Design review of the part built by this model. Coordinates are the model's own, in mm. Face numbers are marked on the shaded views. A direction names the side the tool comes from. Give positions to 0.01 mm unless a question says otherwise; leave off trailing zeros. Write each loop counter-clockwise with the first axis right and the second up, starting at its lowest first coordinate (ties: lowest second). Pieces come first, ordered by that corner, then holes. Notation, with made-up numbers: M 88,18.25 L 129,18.25 A35 ccw 129,56.25 Z; hole C 5.5,-5.5 d1. An arc over 180 degrees is marked long. One line per item, written item: value. Start each with the question number.
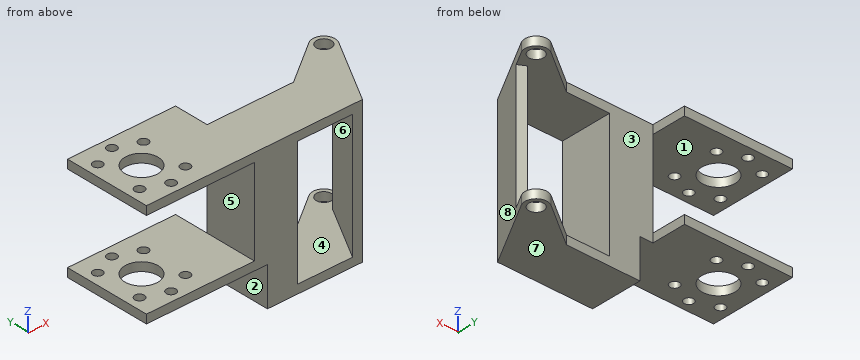
Autodesk Inventor part; units mm, degrees
ref_plane "YZ Plane" through (0, 0, 0) normal (1, 0, 0) x (0, 1, 0)
ref_plane "XZ Plane" through (0, 0, 0) normal (0, 1, 0) x (-1, 0, 0)
ref_plane "XY Plane" through (0, 0, 0) normal (0, 0, 1) x (1, 0, 0)
sketch "Sketch1" plane through (0, 0, 0) normal (0, 1, 0) x (-1, 0, 0)
  line L0 (10.16, 20.955) -> (-21.59, 20.955)
  line L1 (-21.59, 20.955) -> (-21.59, 18.415)
  line L2 (-21.59, 18.415) -> (10.16, 18.415)
  line L3 (10.16, 18.415) -> (10.16, 20.955)
  line L4 (10.16, -6.985) -> (-21.59, -6.985)
  line L5 (-21.59, -6.985) -> (-21.59, -9.525)
  line L6 (-21.59, -9.525) -> (10.16, -9.525)
  line L7 (10.16, -9.525) -> (10.16, -6.985)
  point P0 (0, 0)
  dimension "d0" = 31.75
  dimension "d1" = 2.54
  dimension "d2" = 10.16
  dimension "d3" = 20.955
  dimension "d4" = 31.75
  dimension "d5" = 2.54
  dimension "d6" = 10.16
  dimension "d7" = 30.48
extrude "Extrusion1" add sketch "Sketch1" along normal blind 25.4
sketch "Sketch2" plane through (0, 0, 0) normal (0, 1, 0) x (-1, 0, 0)
  line L0 (-21.59, 18.415) -> (10.16, 18.415)
  line L1 (10.16, -6.985) -> (-21.59, -6.985)
  line L2 (-21.59, 18.415) -> (-34.29, 18.415)
  line L3 (10.16, 18.415) -> (10.16, 20.955)
  line L4 (-21.59, -9.525) -> (-25.4, -9.525)
  line L5 (-21.59, -6.985) -> (-21.59, -9.525)
  line L6 (-21.59, -9.525) -> (-21.59, 18.415)
  line L7 (-25.4, -9.525) -> (-25.4, -20.955)
  line L8 (-25.4, -20.955) -> (-34.29, -20.955)
  line L9 (-34.29, -20.955) -> (-34.29, 18.415)
  line L10 (-21.59, 18.415) -> (10.16, 18.415)
  line L11 (10.16, -9.525) -> (10.16, -6.985)
  line L12 (10.16, 20.955) -> (-21.59, 20.955)
  point P0 (0, 0)
  point P1 (-21.59, -6.985)
  dimension "d16" = 35.56
  dimension "d17" = 41.91
  dimension "d18" = 12.7
extrude "Extrusion2" add sketch "Sketch2" along normal blind 15.24
sketch "Sketch4" plane through (0, 0, 0) normal (0, 1, 0) x (-1, 0, 0)
  line L0 (-34.29, -20.955) -> (-25.4, -20.955)
  line L1 (-34.29, -20.955) -> (-53.34, -20.955)
  line L2 (-53.34, -20.955) -> (-53.34, -18.415)
  line L3 (-53.34, -18.415) -> (-34.29, -18.415)
  line L4 (-34.29, -18.415) -> (-34.29, -20.955)
  line L5 (-21.59, 20.955) -> (-53.34, 20.955)
  line L6 (-53.34, 20.955) -> (-53.34, 18.415)
  line L7 (-53.34, 18.415) -> (-21.59, 18.415)
  line L8 (-21.59, 18.415) -> (-21.59, 20.955)
  line L9 (10.16, 18.415) -> (10.16, 20.955)
  line L10 (10.16, -9.525) -> (10.16, -6.985)
  point P0 (0, 0)
  point P1 (-50.8, -18.415)
  dimension "d20" = 2.54
  dimension "d24" = 2.54
  dimension "d55" = 63.5
  dimension "d56" = 63.5
extrude "Extrusion3" add sketch "Sketch4" along normal blind 15.24
sketch "Sketch5" plane through (-10.16, 25.4, 20.955) normal (0, 0, 1) x (1, 0, 0)
  circle A0 centre (10.16, -12.7) radius 4.8895
  line L0 (0, -25.4) -> (0, 0)
  line L1 (-16.3, -25.4) -> (92.4658, -25.4)
  circle A1 centre (10.16, -22.225) radius 1.397
  circle A2 centre (16.8952, -19.4352) radius 1.397
  circle A3 centre (19.685, -12.7) radius 1.397
  circle A4 centre (16.8952, -5.9648) radius 1.397
  circle A5 centre (10.16, -3.175) radius 1.397
  circle A6 centre (3.4248, -5.9648) radius 1.397
  circle A7 centre (0.635, -12.7) radius 1.397
  circle A8 centre (3.4248, -19.4352) radius 1.397
  point P0 (10.16, -25.4)
  dimension "d26" = 9.779
  dimension "d27" = 10.16
  dimension "d28" = 12.7
  dimension "d29" = 2.794
  dimension "d30" = 9.525
  dimension "d33" = 360
extrude "Extrusion4" cut sketch "Sketch5" against normal through all contours A0 | A1 | A2 | A4 | A5 | A6 | A8
sketch "Sketch6" plane through (-10.16, 25.4, 20.955) normal (0, 0, 1) x (1, 0, 0)
  circle A0 centre (72.3186, -3.302) radius 2.2
  circle A1 centre (10.16, -12.7) radius 4.8895 construction
  line L0 (0, 0) -> (31.75, 0) construction
  line L1 (75.6206, -25.4) -> (75.6206, 0) construction
  line L2 (75.6206, -25.4) -> (101.0206, -25.4) construction
  arc A2 (75.1858, -4.9396) -> (70.3884, -0.6228) centre (72.3186, -3.302) ccw
  line L3 (63.5, -25.4) -> (44.45, -25.4) construction
  line L4 (75.1858, -4.9396) -> (98.796, -4.9396) construction
  line L5 (70.3884, -0.6228) -> (57.15, -10.16)
  line L6 (63.5, -10.16) -> (44.45, -10.16) construction
  line L7 (63.5, -25.4) -> (63.5, -10.16) construction
  line L8 (31.75, -10.16) -> (63.5, -10.16)
  line L9 (0, -25.4) -> (63.5, -25.4)
  line L10 (75.1858, -4.9396) -> (63.5, -25.4)
  line L11 (57.15, -10.16) -> (63.5, -25.4)
  point P0 (10.16, -25.4)
  point P1 (60.96, -25.4)
  point P2 (60.96, -10.16)
  dimension "d37" = 4.4
  dimension "d38" = 62.865
  dimension "d39" = 3.302
  dimension "d40" = 25.4
  dimension "d41" = 90
  dimension "d42" = 3.302
  dimension "d53" = 6.604
  dimension "d57" = 6.35
extrude "Extrusion8" add sketch "Sketch6" against normal blind 2.54
sketch "Sketch9" plane through (25.4, 0, -20.955) normal (0, 0, -1) x (-1, 0, 0)
  line L0 (-39.6182, 20.447) -> (-27.94, 0.2198)
  line L1 (-21.59, 15.24) -> (-34.8284, 24.7772)
  arc A0 (-34.8284, 24.7772) -> (-39.6258, 20.4604) centre (-36.7586, 22.098) ccw
  circle A1 centre (-36.7586, 22.098) radius 2.2
  line L2 (-39.6258, 20.4604) -> (-27.94, 0)
  line L3 (-27.94, 0) -> (-8.89, 0)
  line L4 (-21.59, 15.24) -> (-27.94, 0)
  point P0 (25.4, 0)
extrude "Extrusion10" add sketch "Sketch9" against normal blind 2.54
sketch "Sketch10" plane through (34.29, 0, 18.415) normal (0, 0, -1) x (-1, 0, 0)
  line L0 (-19.05, 0) -> (-30.7358, 20.4604)
  line L1 (-28.2164, 16.0491) -> (-26.0108, 17.3089)
  circle A0 centre (-27.8686, 22.098) radius 2.2 construction
  line L2 (44.45, 0) -> (-19.05, 0) construction
  line L3 (-19.05, 0) -> (-17.5875, 0) construction
  line L4 (-26.0108, 17.3089) -> (-16.1249, 0)
  line L5 (-16.1249, 0) -> (-19.05, 0)
  point P0 (34.29, 0)
  dimension "d64" = 2.54
  dimension "d65" = 5.08
extrude "Extrusion11" add sketch "Sketch10" along normal up to surface (36.83 mm away)
equation "\"d5\" = d1"
equation "\"d56\" = d55"
properties part number "Odometry holder for metal drive train"
Q1. Take a section at B-B, the plane z = -5. Give the boundary of the cut face in (x, y), then the cut area to 3 significant figures.
Q2. For P1, Ø7.5, axis at x = 4, y = 8.5, coming from the -Z side (3 decimals); P2, Ø6, axis at y = 3, z = 12, coming from the +X side; P3, Ø3, axis at x = 6.74, y = 5.96, coming from the +Z side (3 decimals); P4, Ø1.7, axis at x = -6.74, y = 5.96, coming from the -Z side, all flat-tipped, find the tip position at first contact; note any pin that passes through.
Q3. Wall thickness on line 1 (Y direction, x = 0, z = 20.25); line 2 (Z direction, x = 55, y = 10) (3 decimals); line 3 (Z direction, x = 13, y = 20.5) (3 decimals): over which ranges is each line inside the solid? List them lowest first. Write a range as from..to.
Q4. Take a section at A-A, the plane x = 0. State how many separate pieces and enclosed holes the cut face has, then the cut area to 3 significant figures.
Q5. Take a section at D-D, the plane x = 49.5. Give the boundary of the cut face in (y, z) (3 decimals), then the cut area to 3 significant figures.
Q6. Take a section at C-C, the plane y = 12.7. Give the boundary of the cut face in (x, z) (1 decimal), then the cut area to 3 significant figures.
Q7. Machinability: for the marked faces 1, 2, 3 and 4, which of the approach directions +Z, -Z, +X, -X, +Y, -Y give a long, thin tool a straight path to every point of the face, cutting with its end or side? Answer none if there is none.
Q8. The part is to be moulded in two halves that separate along Z. For the marked faces 5, 6, 7 and 8, say which applies: pulls with the +Z half, pulls with the -Z half, needs draft (parallel to the pull), parting line crosses it, or undercut.
Results list:
1. outline: M 21.59,0 L 34.29,0 L 34.29,15.24 L 21.59,15.24 Z; M 50.41,0 L 53.34,0 L 62.51,16.05 L 60.3,17.31 Z
1. area: 242 mm^2
2. P1: stops at z = -9.525
2. P2: stops at x = 56.77
2. P3: stops at z = 20.955
2. P4: passes through
3. line 1: y = 0..1.78, 4.57..7.81, 17.59..20.83, 23.62..25.4
3. line 2: z = -20.955..-18.415, 18.415..20.955
3. line 3: z = -9.525..-6.985, 18.415..20.955
4. separate pieces: 8
4. enclosed holes: 0
4. area: 51.0 mm^2
5. outline: M 0,-20.955 L 17.048,-20.955 L 17.048,-18.415 L 0,-18.415 Z; M 0,18.415 L 17.048,18.415 L 17.048,20.955 L 0,20.955 Z
5. area: 86.6 mm^2
6. outline: M -10.2,-9.5 L -4.9,-9.5 L -4.9,-7 L -10.2,-7 Z; M -10.2,18.4 L -4.9,18.4 L -4.9,21 L -10.2,21 Z; M 4.9,-9.5 L 25.4,-9.5 L 25.4,-21 L 60.6,-21 L 60.6,21 L 4.9,21 L 4.9,18.4 L 21.6,18.4 L 21.6,-7 L 4.9,-7 Z; hole M 34.3,-18.4 L 57.7,-18.4 L 57.7,18.4 L 34.3,18.4 Z
6. area: 842 mm^2
7. face 1: -X, +Y, -Y
7. face 2: -Z, -X, +Y, -Y
7. face 3: +Z, -Z, +Y
7. face 4: +Y
8. face 5: undercut
8. face 6: undercut
8. face 7: pulls with the -Z half
8. face 8: needs draft
